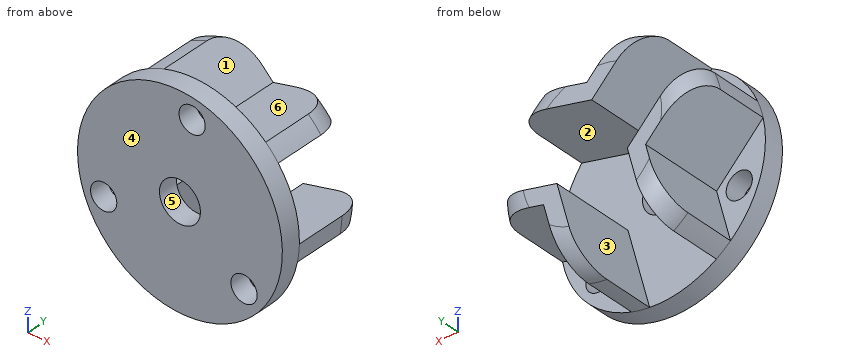
```python
from build123d import *

# Parameters (mm, degrees)
SKETCH1_R           = 62.5
BOSS_EXTRUDE1_DEPTH = 12
BOSS_EXTRUDE2_DEPTH = 50
FILLET1_R           = 20
SKETCH3_R           = 12.5
CUT_EXTRUDE1_DEPTH  = 50
SKETCH4_R           = 8
CUT_EXTRUDE2_DEPTH  = 50


with BuildPart() as part:
    # Sketch1 → Boss-Extrude1 (new body)
    with BuildSketch(Plane(origin=(0, 0, 0), x_dir=(1, 0, 0), z_dir=(0, 1, 0))):
        with Locations(Location((0, 0, 0), (0, 0, 270))):
            Circle(SKETCH1_R)
    extrude(amount=BOSS_EXTRUDE1_DEPTH)

    # Sketch2 → Boss-Extrude2 (add)
    with BuildSketch(Plane(origin=(0, 12, 0), x_dir=(1, 0, 0), z_dir=(0, 1, 0))):
        with BuildLine():
            ThreePointArc((19.168323988, 59.488026993), (13.716019775, 60.976395446), (8.151554557, 61.96613719))
            Line((8.151554557, 61.96613719), (21.395866241, 12.537693074))
            Line((21.395866241, 12.537693074), (62.481297287, 1.528885005))
            ThreePointArc((62.481297287, 1.528885005), (62.119144902, 6.889255161), (61.297971235, 12.198718069))
            Line((61.297971235, 12.198718069), (29.560832051, 20.702658884))
            Line((29.560832051, 20.702658884), (19.168323988, 59.488026993))
        make_face()
        with BuildLine():
            ThreePointArc((41.933980603, -46.344269018), (45.9490976, -42.366619287), (49.588471703, -38.042521922))
            Line((49.588471703, -38.042521922), (0.160027587, -24.798210238))
            Line((0.160027587, -24.798210238), (-29.91659539, -54.874833214))
            ThreePointArc((-29.91659539, -54.874833214), (-25.093302468, -57.241385127), (-20.084585876, -59.184959324))
            Line((-20.084585876, -59.184959324), (3.148612494, -35.951760955))
            Line((3.148612494, -35.951760955), (41.933980603, -46.344269018))
        make_face()
        with BuildLine():
            ThreePointArc((-61.102304591, -13.143757975), (-59.665117375, -18.609776159), (-57.74002626, -23.923615268))
            Line((-57.74002626, -23.923615268), (-21.555893828, 12.260517164))
            Line((-21.555893828, 12.260517164), (-32.564701897, 53.345948209))
            ThreePointArc((-32.564701897, 53.345948209), (-37.025842434, 50.352129966), (-41.213385359, 46.986241255))
            Line((-41.213385359, 46.986241255), (-32.709444544, 15.249102071))
            Line((-32.709444544, 15.249102071), (-61.102304591, -13.143757975))
        make_face()
    extrude(amount=BOSS_EXTRUDE2_DEPTH)

    # Fillet1
    # the kernel refuses this fillet: 20 mm, written as the material it takes off along each edge
    with BuildSketch(Plane(origin=(0, 62, 0), x_dir=(0.24928364261100788, 0, -0.9684305166229467), z_dir=(0.9684305166229467, 0, 0.24928364261100788))) as fillet1_piece_1:
        with BuildLine():
            CenterArc((62.5 - FILLET1_R, -FILLET1_R), FILLET1_R, 0, 90)
            Line((62.5 - FILLET1_R, 0), (62.5, 0))
            Line((62.5, 0), (62.5, -FILLET1_R))
        make_face()
    revolve(axis=Axis((0, 62, 0), (0, 1, 0)), revolution_arc=101.527179198, mode=Mode.SUBTRACT)
    with BuildSketch(Plane(origin=(0, 62, 0), x_dir=(-0.8319838819593003, 0, -0.5547998018744537), z_dir=(0.5547998018744537, 0, -0.8319838819593003))) as fillet1_piece_2:
        with BuildLine():
            CenterArc((62.5 - FILLET1_R, -FILLET1_R), FILLET1_R, 0, 90)
            Line((62.5 - FILLET1_R, 0), (62.5, 0))
            Line((62.5, 0), (62.5, -FILLET1_R))
        make_face()
    revolve(axis=Axis((0, 62, 0), (0, 1, 0)), revolution_arc=102.039649765, mode=Mode.SUBTRACT)
    with BuildSketch(Plane(origin=(0, 62, 0), x_dir=(-0.9633272505010871, 0, 0.26832929106233594), z_dir=(-0.26832929106233594, 0, -0.9633272505010871))) as fillet1_piece_3:
        with BuildLine():
            CenterArc((62.5 - FILLET1_R, -FILLET1_R), FILLET1_R, 0, 90)
            Line((62.5 - FILLET1_R, 0), (62.5, 0))
            Line((62.5, 0), (62.5, -FILLET1_R))
        make_face()
    revolve(axis=Axis((0, 62, 0), (0, 1, 0)), revolution_arc=101.527179198, mode=Mode.SUBTRACT)
    with BuildSketch(Plane(origin=(0, 62, 0), x_dir=(-0.06447878145815908, 0, 0.9979190782531773), z_dir=(-0.9979190782531773, 0, -0.06447878145815908))) as fillet1_piece_4:
        with BuildLine():
            CenterArc((62.5 - FILLET1_R, -FILLET1_R), FILLET1_R, 0, 90)
            Line((62.5 - FILLET1_R, 0), (62.5, 0))
            Line((62.5, 0), (62.5, -FILLET1_R))
        make_face()
    revolve(axis=Axis((0, 62, 0), (0, 1, 0)), revolution_arc=102.039649765, mode=Mode.SUBTRACT)
    with BuildSketch(Plane(origin=(0, 62, 0), x_dir=(0.8964626634174491, 0, -0.443119276378825), z_dir=(0.443119276378825, 0, 0.8964626634174491))) as fillet1_piece_5:
        with BuildLine():
            CenterArc((62.5 - FILLET1_R, -FILLET1_R), FILLET1_R, 0, 90)
            Line((62.5 - FILLET1_R, 0), (62.5, 0))
            Line((62.5, 0), (62.5, -FILLET1_R))
        make_face()
    revolve(axis=Axis((0, 62, 0), (0, 1, 0)), revolution_arc=102.039649765, mode=Mode.SUBTRACT)
    with BuildSketch(Plane(origin=(0, 62, 0), x_dir=(0.7140436078899985, 0, 0.7001012255605856), z_dir=(-0.7001012255605856, 0, 0.7140436078899985))) as fillet1_piece_6:
        with BuildLine():
            CenterArc((62.5 - FILLET1_R, -FILLET1_R), FILLET1_R, 0, 90)
            Line((62.5 - FILLET1_R, 0), (62.5, 0))
            Line((62.5, 0), (62.5, -FILLET1_R))
        make_face()
    revolve(axis=Axis((0, 62, 0), (0, 1, 0)), revolution_arc=101.527179198, mode=Mode.SUBTRACT)

    # Sketch3 → Cut-Extrude1 (cut)
    with BuildSketch(Plane(origin=(0, 12, 0), x_dir=(1, 0, 0), z_dir=(0, 1, 0))):
        with Locations(Location((0, 0, 0), (0, 0, 270))):
            Circle(SKETCH3_R)
    extrude(amount=-CUT_EXTRUDE1_DEPTH, mode=Mode.SUBTRACT)

    # Sketch4 → Cut-Extrude2 (cut)
    with BuildSketch(Plane(origin=(0, 12, 0), x_dir=(1, 0, 0), z_dir=(0, 1, 0))):
        with Locations(Location((39.110778617, 31.150393192, 0), (0, 0, 270))):
            Circle(SKETCH4_R)
        with Locations(Location((7.421642534, -49.44612444, 0), (0, 0, 270))):
            Circle(SKETCH4_R)
        with Locations(Location((-46.53242115, 18.295731248, 0), (0, 0, 270))):
            Circle(SKETCH4_R)
    extrude(amount=-CUT_EXTRUDE2_DEPTH, mode=Mode.SUBTRACT)


solid = part.part
```
Geometry check sheet. Reference: the model listing, model coordinates, mm. Face numbers are marked on the shaded views. A direction names the side the tool comes from. Round coordinates to 2 decimals unless told otherwise and drop trailing zeros. Order: outer loops, then holes, each group sorted by start corner. A loop starts at its lowest first (then second) coordinate and runs counter-clockwise, first axis right, second up. Notation, with made-up numbers: M 87,37.5 L 92,37.5 A32 cw 92,70.5 Z; hole C 4,83.25 d7. An arc over 180 degrees is marked long. Answer as CSV lines item,"result".
1) Sectioned sample at C-C on y = 9. Record the cut outline in (x, z), and give its area (3 significant figures).
Entries:
outline,"C 0,0 d125; hole C -46.53,-18.3 d16; hole C 0,0 d25; hole C 7.42,49.45 d16; hole C 39.11,-31.15 d16"
area,"11,200 mm2"
2) Sectioned sample at B-B on z = 0. Record the cut outline in (x, y).
Entries:
outline,"M -62.5,0 L -12.5,0 L -12.5,12 L -33.82,12 L -33.82,62 L -42.5,62 A20 ccw -47.96,61.24 L -47.96,12 L -62.5,12 Z; M 12.5,0 L 62.5,0 L 62.5,12 L 12.5,12 Z"
3) Gauge pin test, flat ends, axial feed: pin 1 Ø8 at (y, z) = (35, -41) entering from +X; pin 2 Ø10 at (x, z) = (34.5, 25) entering from +Y; pin 3 Ø10 at (x, z) = (48, 43.5) entering from +Y. Record the tip position at first contact, or that the pin passes through.
Entries:
pin 1,"x = 25.19"
pin 2,"y = 12"
pin 3,"y = 52.07"
4) Mould release check, pull along Z, two halves, no side actions. Record for the marked faces 4, 5 and 6: +Z half, -Z half, draft (parallel to the pull), parting line (faces both ways), or undercut.
Entries:
face 4,"draft"
face 5,"undercut"
face 6,"+Z half"
5) Thickness scan on probe 1 along Y at (x, z) = (5, 23); probe 2 along Y at (x, z) = (37.5, 37); probe 3 along X at (y, z) = (45.5, 48.5). Record the ranges inside material, lowest first. Write a range as [from, to].
Entries:
probe 1,"[0, 12]"
probe 2,"[0, 59.21]"
probe 3,"[-23.54, -9.4]"
6) Sectioned sample at A-A on y = 39.5. Record the cut outline in (x, z).
Entries:
outline,"M -61.1,13.14 L -32.71,-15.25 L -41.21,-46.99 A62.5 ccw -32.56,-53.35 L -21.56,-12.26 L -57.74,23.92 A62.5 ccw Z; M -29.92,54.87 L 0.16,24.8 L 49.59,38.04 A62.5 ccw 41.93,46.34 L 3.15,35.95 L -20.08,59.18 A62.5 ccw Z; M 8.15,-61.97 A62.5 ccw 19.17,-59.49 L 29.56,-20.7 L 61.3,-12.2 A62.5 ccw 62.48,-1.53 L 21.4,-12.54 Z"
7) Tool access check on the marked faces 1, 2 and 3. Record the directions out of +Z, -Z, +X, -X, +Y, -Y that give a thin tool (end or side, any length) a straight path to the whole face; none if there is none.
Entries:
face 1,"+Z, +Y"
face 2,"+X, +Y"
face 3,"+Y"
